Verification items for the finished model (mm, model axes). A direction names the side the tool comes from. Round coordinates to 2 decimals unless told otherwise and drop trailing zeros. Order: outer loops, then holes, each group sorted by start corner. A loop starts at its lowest first (then second) coordinate and runs counter-clockwise, first axis right, second up. Notation, with made-up numbers: M -12.5,34 L 29.5,34 A18 ccw 29.5,69 Z; hole C 59,47 d7. An arc over 180 degrees is marked long. Answer as a JSON object with one key per item and string values. Group by question number.
```python
from build123d import *

# Parameters (mm, degrees)
F0_W     = 20
F0_H     = 17.45
F1_DEPTH = 8
F0_W_2   = 6
F0_H_2   = 6
F0_R     = 1
F2_DEPTH = 1
F3_DEPTH = 24
F4_W     = 6
F4_H     = 6
F5_DEPTH = 1
F6_R     = 1.5
F7_W     = 5
F7_H     = 5
F8_DEPTH = 0.2
F9_R     = 1


with BuildPart() as f1:
    # F0 (on Front) → F1 (new body)
    with BuildSketch(Plane.XZ):
        with Locations((10, 8.725)):
            Rectangle(F0_W, F0_H)
        Polygon((19, 16.45), (19, 11.225), (19, 6.225), (19, 1), (1, 1), (1, 16.45), align=None, mode=Mode.SUBTRACT)
    extrude(amount=F1_DEPTH)

    # F0 (on Front) → F2 (join)
    with BuildSketch(Plane.XZ):
        Polygon((19, 11.225), (14, 11.225), (14, 15.225), (2, 15.225), (2, 11.725), (8, 11.725), (8, 5.725), (2, 5.725), (2, 2.225), (14, 2.225), (14, 6.225), (19, 6.225), align=None)
        with Locations((5, 8.725)):
            Rectangle(F0_W_2, F0_H_2)
        with Locations((5, 8.725)):
            Circle(F0_R, mode=Mode.SUBTRACT)
    extrude(amount=F2_DEPTH)

    # F0 (on Front) → F3 (join)
    with BuildSketch(Plane.XZ):
        with Locations((5, 8.725)):
            Circle(F0_R)
    extrude(amount=F3_DEPTH)

    # F4 (on face) → F5 (join)
    with BuildSketch(Plane.XZ.offset(24)):
        with Locations((5, 8.725)):
            Rectangle(F4_W, F4_H)
    extrude(amount=-F5_DEPTH)

    # F6
    f6_edges = [f1.edges().sort_by_distance(p)[0] for p in [
        (4, -23, 8.725),
        (4, -1, 8.725),
    ]]
    fillet(f6_edges, radius=F6_R)

    # F7 (on face) → F8 (cut)
    with BuildSketch(Plane.XZ.offset(1)):
        with Locations((16.5, 8.725)):
            Rectangle(F7_W, F7_H)
    extrude(amount=-F8_DEPTH, mode=Mode.SUBTRACT)

    # F9
    f9_edges = [f1.edges().sort_by_distance(p)[0] for p in [
        (2, -0.5, 15.225),
        (14, -0.5, 15.225),
        (2, -0.5, 2.225),
        (14, -0.5, 2.225),
    ]]
    fillet(f9_edges, radius=F9_R)


solid = f1.part
```
Q1. Cross-section at A-A, the plane x = 5. Record the cut outline in (y, z) (3 decimals).
Q2. Tool access check on faces 5 (the face through (16, -0.8, 9)), 6 (the face through (8, -23.5, 8.7)), 7 (the face through (8.1, -0.5, 15.225)), 8 (the face through (5, -23.5, 5.725)), 9 (the face through (5, -23.5, 11.725)). Record the directions out of +Z, -Z, +X, -X, +Y, -Y that give a thin tool (end or side, any length) a straight path to the whole face; none if there is none.
Q3. Cross-section at B-B, the plane x = 12.25. Record the cut outline in (y, z) (3 decimals), then the cut area to 3 significant figures.
Q4. Thickness scan on line 1 (Z direction, x = 13, y = -3); line 2 (X direction, y = -3.75, z = 12.75); line 3 (Y direction, x = 10.75, z = 12.75). Record the ranges inside material, lowest first. Write a range as from..to.
Q5. Gauge pin test, flat ends, axial feed: pin 1 Ø2.5 at (x, z) = (17.5, 8.5) entering from -Y; pin 2 Ø0.8 at (y, z) = (-23.5, 8) entering from +X; pin 3 Ø1.1 at (y, z) = (-23.5, 9) entering from -X. Record the tip position at first contact, or that the pin passes through.
Q6. Release check for a two-part mould opening along Y. For faces 1 (the face through (5, -24, 9)), 2 (the face through (4.78, -11.87, 7.75)), 3 (the face through (8, 0, 11)), 4 (the face through (7.9, -0.5, 2.225)) record: released by +Y, released by -Y, zero draft, split by the parting line, or undercut.
Q7. Cross-section at C-C, the plane y = -17.25. Record the cut outline in (x, z) (3 decimals), then the cut area to 3 significant figures.
Conclusion:
{
 "1": {"outline": "M -24,5.725 L -23,5.725 L -23,6.225 A1.5 cw -21.5,7.725 L -2.5,7.725 A1.5 cw -1,6.225 L -1,2.225 L 0,2.225 L 0,15.225 L -1,15.225 L -1,11.225 A1.5 cw -2.5,9.725 L -21.5,9.725 A1.5 cw -23,11.225 L -23,11.725 L -24,11.725 Z; M -8,0 L 0,0 L 0,1 L -8,1 Z; M -8,16.45 L 0,16.45 L 0,17.45 L -8,17.45 Z"},
 "2": {"face 5": "-Y", "face 6": "+Z, -Z, +X, -Y", "face 7": "+Y, -Y", "face 8": "-Z, +X, -X, -Y", "face 9": "+Z, +X, -X, -Y"},
 "3": {"outline": "M -8,0 L 0,0 L 0,1 L -8,1 Z; M -8,16.45 L 0,16.45 L 0,17.45 L -8,17.45 Z; M -1,2.225 L 0,2.225 L 0,15.225 L -1,15.225 Z", "area": "29.0 mm2"},
 "4": {"line 1": "0..1, 16.45..17.45", "line 2": "0..1, 19..20", "line 3": "-1..0"},
 "5": {"pin 1": "y = -0.8", "pin 2": "x = 8", "pin 3": "x = 2"},
 "6": {"face 1": "released by -Y", "face 2": "undercut", "face 3": "released by +Y", "face 4": "zero draft"},
 "7": {"outline": "C 5,8.725 d2", "area": "3.14 mm2"}
}
